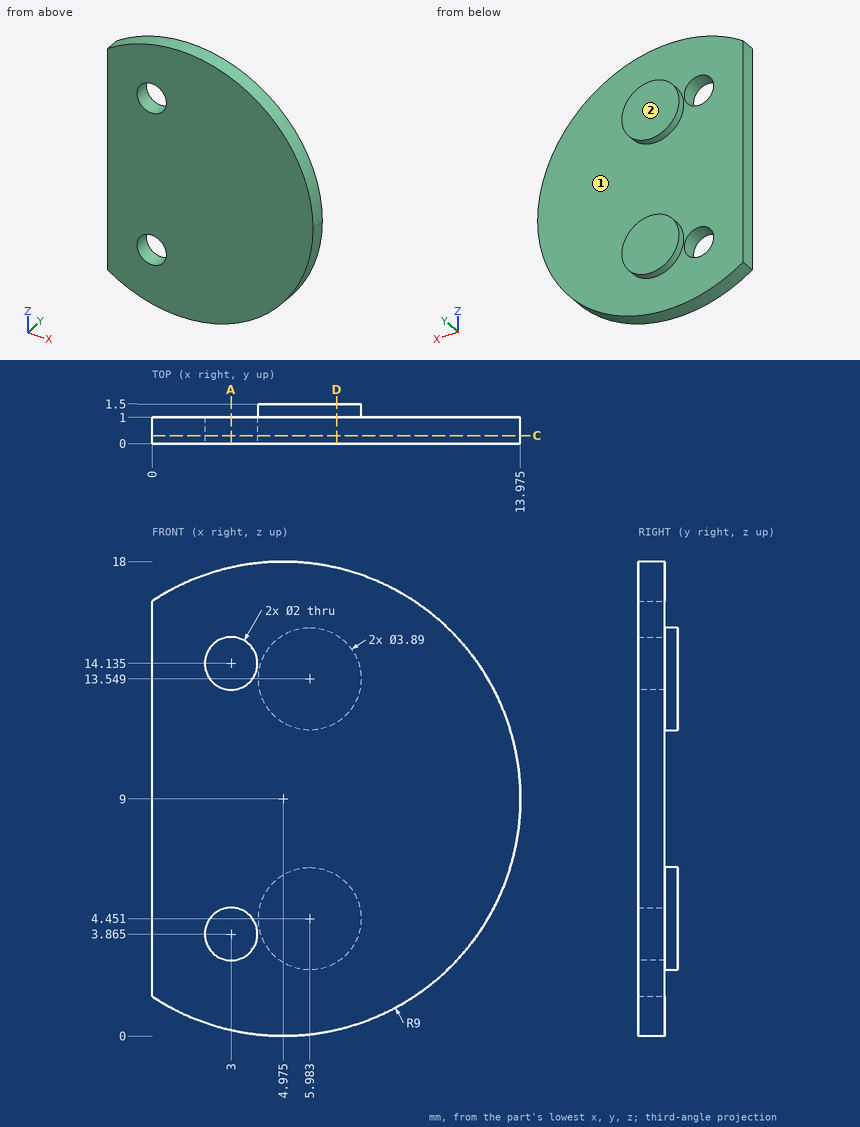
Check sheet for the drawn part. Datum: minimum x, y, z corner. Units: mm. A direction names the side the tool comes from. Round coordinates to 2 decimals unless told otherwise and drop trailing zeros. Order: outer loops, then holes, each group sorted by start corner. A loop starts at its lowest first (then second) coordinate and runs counter-clockwise, first axis right, second up. Notation, with made-up numbers: (58.25, 2.5) -> (71.25, 2.5) arc R14 ccw to (71.25, 15.5) -> close; hole circle Ø5 at (55, 45.25). An arc over 180 degrees is marked (long way). Return JSON: item names as keys, results as strings. Group by question number.
Q1. Tool access check on the marked faces 1 and 2. Record the directions out of +Z, -Z, +X, -X, +Y, -Y that give a thin tool (end or side, any length) a straight path to the whole face; none if there is none.
Q2. Section check D-D, the plane x = 7. Record the boundary of the cut face in (y, z).
Q3. Section check A-A, the plane x = 3. Record the boundary of the cut face in (y, z) (1 decimal).
Q4. Section check C-C, the plane y = 0.3. Record the boundary of the cut face in (x, z) (1 decimal).
Q5. Material ranges on probe 1 along X at (y, z) = (0.65, 14); probe 2 along Y at (x, z) = (11.75, 14.5); probe 3 along Z at (x, y) = (5.75, 1.1), recorded low to high. Write a range as from..to.
Q6. Gauge pin test, flat ends, axial feed: pin 1 (4 mm diameter, centred on x = 2, z = 7.5, fed in from +Y); pin 2 (8 mm diameter, centred on x = 10, z = 10, fed in from +Y). Record the tip position at first contact, or that the pin passes through.
Numbers:
{
 "1": {"face 1": "+Y", "face 2": "+Z, -Z, +X, -X, +Y"},
 "2": {"outline": "(0, 0.23) -> (1, 0.23) -> (1, 2.79) -> (1.5, 2.79) -> (1.5, 6.11) -> (1, 6.11) -> (1, 11.89) -> (1.5, 11.89) -> (1.5, 15.21) -> (1, 15.21) -> (1, 17.77) -> (0, 17.77) -> close"},
 "3": {"outline": "(0, 0.2) -> (1, 0.2) -> (1, 2.9) -> (0, 2.9) -> close; (0, 4.9) -> (1, 4.9) -> (1, 13.1) -> (0, 13.1) -> close; (0, 15.1) -> (1, 15.1) -> (1, 17.8) -> (0, 17.8) -> close"},
 "4": {"outline": "(0, 1.5) arc R9 ccw (long way) to (0, 16.5) -> close; hole circle Ø2 at (3, 3.9); hole circle Ø2 at (3, 14.1)"},
 "5": {"probe 1": "0..2.01, 3.99..12.46", "probe 2": "0..1", "probe 3": "2.52..6.38, 11.62..15.48"},
 "6": {"pin 1": "y = 1", "pin 2": "y = 1.5"}
}
